The listing builds one solid part. Answer for the finished solid, in the listing's coordinates (mm). A direction names the side the tool comes from. Round coordinates to 2 decimals unless told otherwise and drop trailing zeros. Write each loop counter-clockwise with the first axis right and the second up, starting at its lowest first coordinate (ties: lowest second). Pieces come first, ordered by that corner, then holes. Notation, with made-up numbers: (73.5, 85.5) - (94.5, 85.5) arc R21 cw to (94.5, 114.5) - close; hole circle Ø11 at (58, 68.5). An arc over 180 degrees is marked (long way). Answer as CSV lines item,"result". Start each with the question number.
Item 1: A cutting plane is placed at C-C on z = 0. Determine the outline of the cut face in (x, y), and give its area (3 significant figures).
Item 2: Which of the six approach directions +Z, -Z, +X, -X, +Y, -Y give full straight-line access (tool end or side, diameter ignored) to faces 4 (the flat face through (19, 1, 0)), 5 (the conical face through (-21.62, 0.94, 5.86))?
Item 3: For a pull along Y with two mould halves and no side action, classify faces 1 (the conical face through (-21.62, 0.94, -5.86)), 2 (the flat face through (-6.5, -16, 6)), 3 (the flat face through (19, -1, 0)) as pulls with the +Y half, pulls with the -Y half, needs draft (parallel to the pull), parting line crosses it, or undercut.
Item 4: Flat-ended cylindrical pins translate along their axes: pin 1 (2 mm diameter, centred on x = -2, z = -3, fed in from +Y); pin 2 (5.5 mm diameter, centred on x = 19, z = 0, fed in from +Y); pin 3 (3 mm diameter, centred on y = 7, z = -4.5, fed in from +X); pin 4 (10 mm diameter, centred on x = -6.5, y = -6.5, fed in from -Z). Find the tip coordinate at first contact, or state that the pin passes through.
Item 5: Straight lines are drawn through the part: line 1 along Y through (x, z) = (1, 5.5); line 2 along X through (y, z) = (10, -3.75); line 3 along X through (y, z) = (-0.5, 2.25). For each, find the intervals that lie inside material, in ascending order. Write a range as [from, to].
Item 6: A cutting plane is placed at A-A on x = 0. Determine the outline of the cut face in (y, z), and give its area (3 significant figures).
Item 7: A cutting plane is placed at B-B on z = 3. Determine the outline of the cut face in (x, y), and give its area (3 significant figures).
```python
from build123d import *

# Parameters (mm, degrees)
F2_W     = 10
F2_H     = 2
F3_DEPTH = 12.5
F4_SIZE  = 0.5


with BuildPart() as f1:
    # F0 (on Front) → F1 (revolve)
    with BuildSketch(Plane.XZ):
        with BuildLine():
            Line((-17, -6), (-17, 0))
            Line((-17, 0), (-17, 6))
            Line((-17, 6), (-22, 6))
            Line((-22, 6), (-22, 2))
            ThreePointArc((-22, 2), (-20, 0), (-22, -2))
            Line((-22, -2), (-22, -6))
            Line((-22, -6), (-17, -6))
        make_face()
    revolve(axis=Axis((0, 0, 3.54172), (0, 0, 1)))

    # F2 (on Top) → F3 (cut, symmetric)
    with BuildSketch(Plane.XY):
        with Locations((20, 0)):
            Rectangle(F2_W, F2_H)
    extrude(amount=F3_DEPTH, both=True, mode=Mode.SUBTRACT)

    # F4
    f4_edges = [f1.edges().sort_by_distance(p)[0] for p in [
        (-0.500129, -21.994315, -6),
        (-0.500129, -21.994315, 6),
    ]]
    chamfer(f4_edges, length=F4_SIZE)


solid = f1.part
```
Geometry says:
1,outline,"(16.97, -1) arc R17 cw (long way) to (16.97, 1) - (19.97, 1) arc R20 ccw (long way) to (19.97, -1) - close"
1,area,"343 mm^2"
2,face 4,"+Z, -Z, +X"
2,face 5,"+Z"
3,face 1,"parting line crosses it"
3,face 2,"needs draft"
3,face 3,"undercut"
4,pin 1,"stops at y = 21.98"
4,pin 2,"stops at y = 13.83"
4,pin 3,"stops at x = 21.3"
4,pin 4,"passes through"
5,line 1,"y = [-21.98, -16.97], [16.97, 21.98]"
5,line 2,"x = [-19.6, -13.75], [13.75, 19.6]"
5,line 3,"x = [-21.99, -16.99]"
6,outline,"(-22, -5.5) - (-21.5, -6) - (-17, -6) - (-17, 6) - (-21.5, 6) - (-22, 5.5) - (-22, 2) arc R2 cw to (-22, -2) - close; (17, -6) - (21.5, -6) - (22, -5.5) - (22, -2) arc R2 cw to (22, 2) - (22, 5.5) - (21.5, 6) - (17, 6) - close"
6,area,"107 mm^2"
7,outline,"(16.97, -1) arc R17 cw (long way) to (16.97, 1) - (21.98, 1) arc R22 ccw (long way) to (21.98, -1) - close"
7,area,"603 mm^2"
